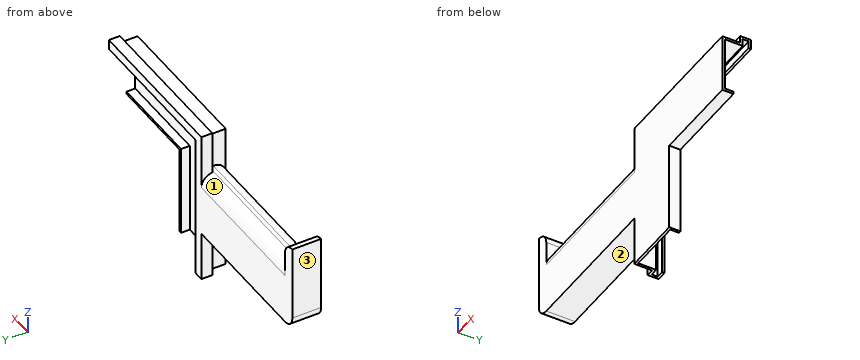
from build123d import *

# Parameters (mm, degrees)
F0_W         = 23.8
F0_H         = 23.8
F0_W_2       = 36.2
F0_H_2       = 36.2
F1_DEPTH     = 1
F2_W         = 59
F2_H         = 1
F2_W_2       = 1
F2_H_2       = 59
F3_DEPTH     = 7.2
F4_W         = 36.2
F4_H         = 1
F5_DEPTH     = 3.5
F6_W         = 60
F6_H         = 1
F7_DEPTH     = 3
F8_W         = 60
F8_H         = 1
F9_DEPTH     = 3.4
F10_W        = 60
F10_H        = 1
F11_DEPTH    = 3
F12_W        = 1
F12_H        = 60
F13_DEPTH    = 3
F14_W        = 1
F14_H        = 60
F15_DEPTH    = 3.4
F16_W        = 1
F16_H        = 60
F17_DEPTH    = 3
F18_DEPTH    = 3
F19_DEPTH    = 2
F20_W        = 7.2
F20_H        = 25.4523856565
F21_DEPTH    = 65
F22_W        = 4.4
F22_H        = 25.4523856565
F23_DEPTH    = 62
F24_W        = 5
F24_H        = 11.6
F25_DEPTH    = 10
F26_R        = 4.99999
F27_T1_DEPTH = 60
F27_T3_DEPTH = 57
F27_T8_DEPTH = 69.5
F28_R        = 5


# Not quite as in the source:
# - a fillet or chamfer that OpenCascade refuses, or shapes differently, is made with other operations: its cross-section is extruded or revolved along the edge and cut away or added
# - a fillet or chamfer is up to 0.001 mm smaller than in the source, because OpenCascade refuses the exact size


with BuildPart() as f1:
    # F0 (on Front) → F1 (new body)
    with BuildSketch(Plane.XZ):
        with Locations((-18.1, 18.1)):
            Rectangle(F0_W, F0_H)
        with Locations((11.9, 18.1)):
            Rectangle(F0_W_2, F0_H)
        with Locations((-18.1, -11.9)):
            Rectangle(F0_W, F0_H_2)
    extrude(amount=F1_DEPTH)

    # F2 (on face) → F3 (join)
    with BuildSketch(Plane(origin=(0, 0, 0), x_dir=(-1, 0, 0), z_dir=(0, 1, 0))):
        with Locations((-0.5, 29.5)):
            Rectangle(F2_W, F2_H)
        with Locations((29.5, 29.5)):
            Rectangle(F2_W_2, F2_H)
        with Locations((29.5, -0.5)):
            Rectangle(F2_W_2, F2_H_2)
    extrude(amount=F3_DEPTH)

    # F4 (on face) → F5 (join)
    with BuildSketch(Plane(origin=(0, 0, 0), x_dir=(-1, 0, 0), z_dir=(0, 1, 0))):
        with Locations((-11.9, 6.7)):
            Rectangle(F4_W, F4_H)
        Polygon((6.2, 7.2), (6.2, 6.2), (6.2, -30), (7.2, -30), (7.2, 7.2), align=None)
    extrude(amount=F5_DEPTH)

    # F6 (on face) → F7 (join)
    with BuildSketch(Plane.XY.offset(30)):
        with Locations((0, 6.7)):
            Rectangle(F6_W, F6_H)
    extrude(amount=F7_DEPTH)

    # F8 (on face) → F9 (join)
    with BuildSketch(Plane(origin=(0, 7.2, 0), x_dir=(-1, 0, 0), z_dir=(0, 1, 0))):
        with Locations((0, 32.5)):
            Rectangle(F8_W, F8_H)
    extrude(amount=F9_DEPTH)

    # F10 (on face) → F11 (join)
    with BuildSketch(Plane(origin=(0, 0, 32), x_dir=(1, 0, 0), z_dir=(0, 0, -1))):
        with Locations((0, -10.1)):
            Rectangle(F10_W, F10_H)
    extrude(amount=F11_DEPTH)

    # F12 (on face) → F13 (join)
    with BuildSketch(Plane(origin=(-30, 0, 0), x_dir=(0, -1, 0), z_dir=(-1, 0, 0))):
        with Locations((-6.7, 0)):
            Rectangle(F12_W, F12_H)
    extrude(amount=F13_DEPTH)

    # F14 (on face) → F15 (join)
    with BuildSketch(Plane(origin=(0, 7.2, 0), x_dir=(-1, 0, 0), z_dir=(0, 1, 0))):
        with Locations((32.5, 0)):
            Rectangle(F14_W, F14_H)
    extrude(amount=F15_DEPTH)

    # F16 (on face) → F17 (join)
    with BuildSketch(Plane.YZ.offset(-32)):
        with Locations((10.1, 0)):
            Rectangle(F16_W, F16_H)
    extrude(amount=F17_DEPTH)

    # F18 (add): a face of the model
    f18_faces = [f1.faces().sort_by_distance(p)[0] for p in [
        (-30, 6.2532541078, 31.5),
    ]]
    extrude(f18_faces, amount=F18_DEPTH)

    # F19 (add): a face of the model
    f19_faces = [f1.faces().sort_by_distance(p)[0] for p in [
        (-32.5, 8.4, 30),
    ]]
    extrude(f19_faces, amount=F19_DEPTH)

    # F20 (on face) → F21 (join)
    with BuildSketch(Plane(origin=(-30, 0, 0), x_dir=(0, -1, 0), z_dir=(-1, 0, 0))):
        with Locations((-2.6, 2.8769155033)):
            Rectangle(F20_W, F20_H)
    extrude(amount=F21_DEPTH)

    # F22 (on face) → F23 (join)
    with BuildSketch(Plane(origin=(-33, 0, 0), x_dir=(0, -1, 0), z_dir=(-1, 0, 0))):
        with Locations((-8.4, 2.8769155033)):
            Rectangle(F22_W, F22_H)
    extrude(amount=F23_DEPTH)

    # F24 (on face) → F25 (join)
    with BuildSketch(Plane.XY.offset(15.6031083316)):
        with Locations((-92.5, 4.8)):
            Rectangle(F24_W, F24_H)
    extrude(amount=F25_DEPTH)

    # F26 (radius 5 in the source; OpenCascade refuses exactly that, so slightly less here)
    f26_edges = [f1.edges().sort_by_distance(p)[0] for p in [
        (-90, 4.8, 25.603108),
    ]]
    fillet(f26_edges, radius=F26_R)

    # F27: fillet of radius 5 on 2 edges, made by hand

    # F27_s2 → F27_t1 (cut)
    with BuildSketch(Plane.YZ.offset(-90)):
        with BuildLine():
            ThreePointArc((-1, 10.6031083316), (0.4644660941, 14.1386422375), (4, 15.6031083316))
            Line((4, 15.6031083316), (-1, 15.6031083316))
            Line((-1, 15.6031083316), (-1, 10.6031083316))
        make_face()
    extrude(amount=F27_T1_DEPTH, mode=Mode.SUBTRACT)

    # F27_s4 → F27_t3 (cut)
    with BuildSketch(Plane.YZ.offset(-90)):
        with BuildLine():
            ThreePointArc((5.6, 15.6031083316), (9.1355339059, 14.1386422375), (10.6, 10.6031083316))
            Line((10.6, 10.6031083316), (10.6, 15.6031083316))
            Line((10.6, 15.6031083316), (5.6, 15.6031083316))
        make_face()
    extrude(amount=F27_T3_DEPTH, mode=Mode.SUBTRACT)


with BuildPart() as f27_tool6:
    # F27_s7 → F27_t8 (new body)
    with BuildSketch(Plane.YZ.offset(-20.5)):
        with BuildLine():
            ThreePointArc((5.6, 15.6031083316), (9.1355339059, 14.1386422375), (10.6, 10.6031083316))
            Line((10.6, 10.6031083316), (10.6, 15.6031083316))
            Line((10.6, 15.6031083316), (5.6, 15.6031083316))
        make_face()
    extrude(amount=-F27_T8_DEPTH)

    split(bisect_by=Plane.YZ.offset(-30), keep=Keep.BOTTOM)

    split(bisect_by=Plane.XZ.offset(-6.2), keep=Keep.TOP)


with BuildPart() as f1_1:
    add(f1.part)

    # F27_t5: cut F27_tool6
    add(f27_tool6.part, mode=Mode.SUBTRACT)

    # F28
    f28_edges = [f1_1.edges().sort_by_distance(p)[0] for p in [
        (-95, 4.8, -9.849277),
    ]]
    fillet(f28_edges, radius=F28_R)


solid = f1_1.part
Geometry check sheet. Reference: the model listing, model coordinates, mm. Face numbers are marked on the shaded views. Round coordinates to 2 decimals unless told otherwise and drop trailing zeros. Write each loop counter-clockwise with the first axis right and the second up, starting at its lowest first coordinate (ties: lowest second). Pieces come first, ordered by that corner, then holes.
Item 1: Section check C-C (x = -23). Record the boundary of the cut face in (y, z), plus the area to 3 significant figures.
Determined:
outline: (-1, -30) - (0, -30) - (0, 29) - (7.2, 29) - (7.2, 32) - (9.6, 32) - (9.6, 29) - (10.6, 29) - (10.6, 33) - (6.2, 33) - (6.2, 30) - (-1, 30) - close
area: 76.6 mm2
Item 2: Section check A-A (z = 5). Record the boundary of the cut face in (x, y), plus the area to 3 significant figures.
Determined:
outline: (-95, -1) - (-6.2, -1) - (-6.2, 3.5) - (-7.2, 3.5) - (-7.2, 0) - (-29, 0) - (-29, 7.2) - (-32, 7.2) - (-32, 9.6) - (-29, 9.6) - (-29, 10.6) - (-95, 10.6) - close
area: 785 mm2
Item 3: Section check D-D (z = -21.5). Record the boundary of the cut face in (x, y).
Determined:
outline: (-33, 6.2) - (-30, 6.2) - (-30, -1) - (-6.2, -1) - (-6.2, 3.5) - (-7.2, 3.5) - (-7.2, 0) - (-29, 0) - (-29, 7.2) - (-32, 7.2) - (-32, 9.6) - (-29, 9.6) - (-29, 10.6) - (-33, 10.6) - close
Item 4: Mould release check, pull along X, two halves, no side actions. Record for the marked faces 1, 2 and 3: +X half, -X half, draft (parallel to the pull), parting line (faces both ways), or undercut.
Determined:
face 1: undercut
face 2: draft
face 3: -X half
Item 5: Material ranges on line 1 along Z through (x, y) = (20.5, 2); line 2 along X through (y, z) = (1.25, -19.5); line 3 along X through (y, z) = (8.75, 8.5), recorded low to high.
Determined:
line 1: z = 6.2 to 7.2, 29 to 30
line 2: x = -30 to -29, -7.2 to -6.2
line 3: x = -95 to -32
Item 6: Go/stop test with flat-tipped pins: pin 1 Ø5 at (y, z) = (2, -19.5) entering from +X; pin 2 Ø6 at (x, y) = (-73, 4.5) entering from -Z; pin 3 Ø0.5 at (y, z) = (10, 12) entering from +X. Record where each tip stops, or that it passes through.
Determined:
pin 1: stops at x = -6.2
pin 2: stops at z = -9.85
pin 3: stops at x = -29
